Build history of the part. All positions in model axes, mm. Coordinates: 2 decimals unless noted, no trailing zeros. Loops run counter-clockwise (first coordinate to the right, second up) from the corner with the lowest first, then second, coordinate; pieces in that order, holes last.
Item 1: Drill centre lines: line 1 along Y through (x, z) = (-22.5, 0.65); line 2 along Y through (x, z) = (45, 0.95); line 3 along X through (y, z) = (-25, 1.1). Where is each one in solid material? Low to high.
Item 2: Flat gauge pin, fed straight in: pin 1 (1.8 mm diameter, centred on x = 22.5, y = 38.97, fed in from -Z). Where does the tip first touch, or does it go through?
Item 3: Cut at A-A (x = 45). List the corners of the cut face in (y, z).
Item 4: Cut at D-D (y = 35). List the corners of the cut face in (x, z).
Item 5: Cut at B-B (x = -22.5). List the corners of the cut face in (y, z), and give its area (3 significant figures).
Item 6: Cut at C-C (z = 0.3). List the corners of the cut face in (x, y), and give its area (3 significant figures).
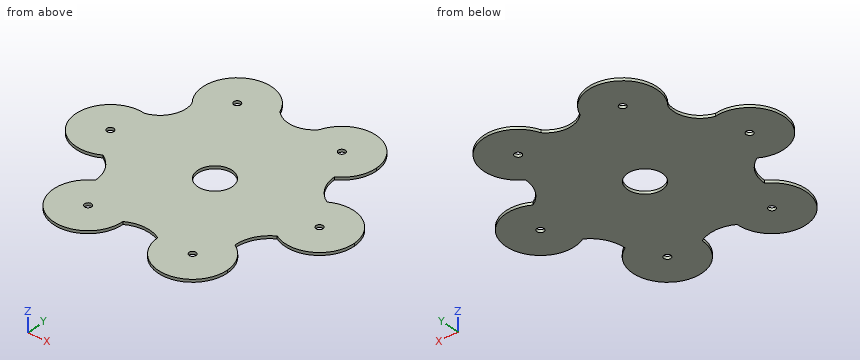
from build123d import *

# Parameters (mm, degrees)
F0_R     = 7.5
F0_R_2   = 1.5
F1_DEPTH = 1.2


with BuildPart() as f1:
    # F0 (on Top) → F1 (new body)
    with BuildSketch(Plane.XY):
        with BuildLine():
            ThreePointArc((-8.441312, 44.201179), (-7.737203, 41.628178), (-7.5, 38.971143))
            ThreePointArc((-7.5, 38.971143), (-17.419662, 24.857669), (-34.058688, 29.41098))
            ThreePointArc((-34.058688, 29.41098), (-35.069793, 20.247554), (-42.5, 14.790199))
            ThreePointArc((-42.5, 14.790199), (-33.543561, 9.682458), (-30, 0))
            ThreePointArc((-30, 0), (-32.009619, -7.5), (-37.5, -12.990381))
            ThreePointArc((-37.5, -12.990381), (-32.009619, -18.480762), (-30, -25.980762))
            ThreePointArc((-30, -25.980762), (-15, -25.980762), (-7.5, -38.971143))
            ThreePointArc((-7.5, -38.971143), (0, -36.961524), (7.5, -38.971143))
            ThreePointArc((7.5, -38.971143), (15, -25.980762), (30, -25.980762))
            ThreePointArc((30, -25.980762), (32.009619, -18.480762), (37.5, -12.990381))
            ThreePointArc((37.5, -12.990381), (30, 0), (37.5, 12.990381))
            ThreePointArc((37.5, 12.990381), (32.009619, 18.480762), (30, 25.980762))
            ThreePointArc((30, 25.980762), (12.817542, 27.514704), (8.441312, 44.201179))
            ThreePointArc((8.441312, 44.201179), (0, 40.495108), (-8.441312, 44.201179))
        make_face()
        Circle(F0_R, mode=Mode.SUBTRACT)
        with BuildLine():
            ThreePointArc((-30, 0), (-33.543561, 9.682458), (-42.5, 14.790199))
            ThreePointArc((-42.5, 14.790199), (-59.762797, -2.657035), (-37.5, -12.990381))
            ThreePointArc((-37.5, -12.990381), (-32.009619, -7.5), (-30, 0))
        make_face()
        with Locations((-45, 0)):
            Circle(F0_R_2, mode=Mode.SUBTRACT)
        with BuildLine():
            ThreePointArc((-34.058688, 29.41098), (-17.419662, 24.857669), (-7.5, 38.971143))
            ThreePointArc((-7.5, 38.971143), (-7.737203, 41.628178), (-8.441312, 44.201179))
            ThreePointArc((-8.441312, 44.201179), (-30, 51.961524), (-34.058688, 29.41098))
        make_face()
        with Locations((-22.5, 38.971143)):
            Circle(F0_R_2, mode=Mode.SUBTRACT)
        with BuildLine():
            ThreePointArc((37.5, 38.971143), (25.157035, 53.73394), (8.441312, 44.201179))
            ThreePointArc((8.441312, 44.201179), (12.817542, 27.514704), (30, 25.980762))
            ThreePointArc((30, 25.980762), (35.490381, 31.471143), (37.5, 38.971143))
        make_face()
        with Locations((22.5, 38.971143)):
            Circle(F0_R_2, mode=Mode.SUBTRACT)
        with BuildLine():
            ThreePointArc((60, 0), (52.5, 12.990381), (37.5, 12.990381))
            ThreePointArc((37.5, 12.990381), (30, 0), (37.5, -12.990381))
            ThreePointArc((37.5, -12.990381), (52.5, -12.990381), (60, 0))
        make_face()
        with Locations((45, 0)):
            Circle(F0_R_2, mode=Mode.SUBTRACT)
        with BuildLine():
            ThreePointArc((37.5, -38.971143), (35.490381, -31.471143), (30, -25.980762))
            ThreePointArc((30, -25.980762), (15, -25.980762), (7.5, -38.971143))
            ThreePointArc((7.5, -38.971143), (22.5, -53.971143), (37.5, -38.971143))
        make_face()
        with Locations((22.5, -38.971143)):
            Circle(F0_R_2, mode=Mode.SUBTRACT)
        with BuildLine():
            ThreePointArc((-7.5, -38.971143), (-15, -25.980762), (-30, -25.980762))
            ThreePointArc((-30, -25.980762), (-30, -51.961524), (-7.5, -38.971143))
        make_face()
        with Locations((-22.5, -38.971143)):
            Circle(F0_R_2, mode=Mode.SUBTRACT)
    extrude(amount=F1_DEPTH)


solid = f1.part
Filled sheet:
1. line 1: y = -53.97 to -40.47, -37.47 to 37.47, 40.47 to 53.97
1. line 2: y = -15 to -1.5, 1.5 to 15
1. line 3: x = -30.03 to 30.03
2. pin 1: passes through
3. outline: (-15, 0) - (-1.5, 0) - (-1.5, 1.2) - (-15, 1.2) - close; (1.5, 0) - (15, 0) - (15, 1.2) - (1.5, 1.2) - close
4. outline: (-36.96, 0) - (36.96, 0) - (36.96, 1.2) - (-36.96, 1.2) - close
5. outline: (-53.97, 0) - (-40.47, 0) - (-40.47, 1.2) - (-53.97, 1.2) - close; (-37.47, 0) - (37.47, 0) - (37.47, 1.2) - (-37.47, 1.2) - close; (40.47, 0) - (53.97, 0) - (53.97, 1.2) - (40.47, 1.2) - close
5. area: 122 mm2
6. outline: (-42.5, 14.79) arc R15 ccw (long way) to (-37.5, -12.99) arc R15 cw to (-30, -25.98) arc R15 ccw (long way) to (-7.5, -38.97) arc R15 cw to (7.5, -38.97) arc R15 ccw (long way) to (30, -25.98) arc R15 cw to (37.5, -12.99) arc R15 ccw (long way) to (37.5, 12.99) arc R15 cw to (30, 25.98) arc R15 ccw (long way) to (8.44, 44.2) arc R11.47 cw to (-8.44, 44.2) arc R15 ccw (long way) to (-34.06, 29.41) arc R11.47 cw to start; hole circle Ø3 at (-45, 0); hole circle Ø3 at (-22.5, -38.97); hole circle Ø3 at (-22.5, 38.97); hole circle Ø15 at (0, 0); hole circle Ø3 at (22.5, -38.97); hole circle Ø3 at (22.5, 38.97); hole circle Ø3 at (45, 0)
6. area: 7,860 mm2
